The listing builds one solid part. Answer for the finished solid, in the listing's coordinates (mm). Face numbers are marked on the shaded views. Coordinates: 2 decimals unless noted, no trailing zeros. Loops run counter-clockwise (first coordinate to the right, second up) from the corner with the lowest first, then second, coordinate; pieces in that order, holes last. Notation, with made-up numbers: M 73.5,60 L 123.5,60 A20 ccw 123.5,76 Z; hole C 80.25,-10 d4. An arc over 180 degrees is marked long. Return JSON: item names as keys, results as strings. Group by question number.
1. Section C-C (x = 20) is taken. Write down the section's boundary in (y, z).
2. Given P1, Ø2, axis at x = 4, y = -10.5, coming from the +Z side, flat-ended and moving along its own axis, determine where the tip first touches the part or whether it passes through.
3. Section B-B (y = 0) is taken. Write down the section's boundary in (x, z).
4. Section A-A (z = -20) is taken. Write down the section's boundary in (x, y), then the cut area to 3 significant figures.
5. Straight lines are drawn through the part: L1, parallel to Z at x = -20, y = 3; L2, parallel to X at y = 0, z = -8; L3, parallel to Z at x = -21, y = -11.5. For each, find the intervals that lie inside material, in ascending order. Write a range as from..to.
6. Section D-D (x = 0) is taken. Write down the section's boundary in (y, z), then the cut area to 3 significant figures.
7. The mould has two halves that part along Y. Classify the marked faces 1, 2, 3 and 4: pulls with the +Y half, pulls with the -Y half, needs draft (parallel to the pull), parting line crosses it, or undercut.
```python
from build123d import *

# Parameters (mm, degrees)
BOSS_EXTRUDE1_DEPTH      = 40
BOSS_EXTRUDE1_DEPTH_BACK = 30
SKETCH1_W                = 70
SKETCH1_H                = 40
SKETCH1_R                = 10
CUT_EXTRUDE1_DEPTH       = 25
CUT_EXTRUDE1_DEPTH_BACK  = 25
SKETCH2_R                = 4.05
CUT_EXTRUDE2_START       = 40
SKETCH3_R                = 14.35
CUT_EXTRUDE2_DEPTH       = 8.1
CUT_EXTRUDE3_START       = -30
SKETCH4_R                = 14.2875
CUT_EXTRUDE3_DEPTH       = 8.1


with BuildPart() as part:
    # Sketch1 → Boss-Extrude1 (new, two sides: drawn at the far end of the back side and taken through both)
    with BuildSketch(Plane.XY.offset(-BOSS_EXTRUDE1_DEPTH_BACK)):
        Rectangle(SKETCH1_W, SKETCH1_H)
        Circle(SKETCH1_R, mode=Mode.SUBTRACT)
    extrude(amount=BOSS_EXTRUDE1_DEPTH + BOSS_EXTRUDE1_DEPTH_BACK)

    # Sketch2 → Cut-Extrude1 (cut, two sides: drawn at the far end of the back side and taken through both)
    with BuildSketch(Plane(origin=(0, 0, 0), x_dir=(1, 0, 0), z_dir=(0, 1, 0)).offset(-CUT_EXTRUDE1_DEPTH_BACK)):
        with Locations((-20, 20)):
            Circle(SKETCH2_R)
        with Locations((20, 20)):
            Circle(SKETCH2_R)
        with Locations((-20, -20)):
            Circle(SKETCH2_R)
        with Locations((20, -20)):
            Circle(SKETCH2_R)
    extrude(amount=CUT_EXTRUDE1_DEPTH + CUT_EXTRUDE1_DEPTH_BACK, mode=Mode.SUBTRACT)

    # Sketch3 → Cut-Extrude2 (cut)
    with BuildSketch(Plane.XY.offset(CUT_EXTRUDE2_START)):
        Circle(SKETCH3_R)
    extrude(amount=-CUT_EXTRUDE2_DEPTH, mode=Mode.SUBTRACT)

    # Sketch4 → Cut-Extrude3 (cut)
    with BuildSketch(Plane.XY.offset(CUT_EXTRUDE3_START)):
        Circle(SKETCH4_R)
    extrude(amount=CUT_EXTRUDE3_DEPTH, mode=Mode.SUBTRACT)


solid = part.part
```
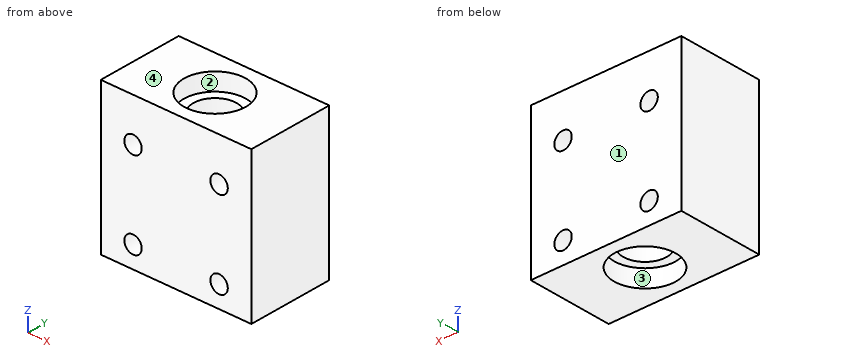
Worked out:
{
 "1": {"outline": "M -20,-30 L 20,-30 L 20,-24.05 L -20,-24.05 Z; M -20,-15.95 L 20,-15.95 L 20,15.95 L -20,15.95 Z; M -20,24.05 L 20,24.05 L 20,40 L -20,40 Z"},
 "2": {"P1": "z = 31.9"},
 "3": {"outline": "M -35,-30 L -14.29,-30 L -14.29,-21.9 L -10,-21.9 L -10,31.9 L -14.35,31.9 L -14.35,40 L -35,40 Z; M 10,-21.9 L 14.29,-21.9 L 14.29,-30 L 35,-30 L 35,40 L 14.35,40 L 14.35,31.9 L 10,31.9 Z; hole C -20,-20 d8.1; hole C -20,20 d8.1; hole C 20,-20 d8.1; hole C 20,20 d8.1"},
 "4": {"outline": "M -35,-20 L -24.05,-20 L -24.05,20 L -35,20 Z; M -15.95,-20 L 15.95,-20 L 15.95,20 L -15.95,20 Z; M 24.05,-20 L 35,-20 L 35,20 L 24.05,20 Z; hole C 0,0 d20", "area": "1,840 mm^2"},
 "5": {"L1": "-30..-24.05, -15.95..15.95, 24.05..40", "L2": "-35..-10, 10..35", "L3": "-30..-23.92, -16.08..16.08, 23.92..40"},
 "6": {"outline": "M -20,-30 L -14.29,-30 L -14.29,-21.9 L -10,-21.9 L -10,31.9 L -14.35,31.9 L -14.35,40 L -20,40 Z; M 10,-21.9 L 14.29,-21.9 L 14.29,-30 L 20,-30 L 20,40 L 14.35,40 L 14.35,31.9 L 10,31.9 Z", "area": "1,260 mm^2"},
 "7": {"face 1": "pulls with the +Y half", "face 2": "undercut", "face 3": "undercut", "face 4": "needs draft"}
}
